Can you work these out from the drawing? Everything is in mm from the part's minimum corner. Coordinates: 2 decimals unless noted, no trailing zeros. Write each loop counter-clockwise with the first axis right and the second up, starting at its lowest first coordinate (ties: lowest second). Pieces come first, ordered by that corner, then holes. Notation, with made-up numbers: M -17.5,28 L 21.5,28 A30 cw 21.5,65 Z; hole C -19,85.5 d2. An arc over 180 degrees is marked long. Write item = value, one per line.
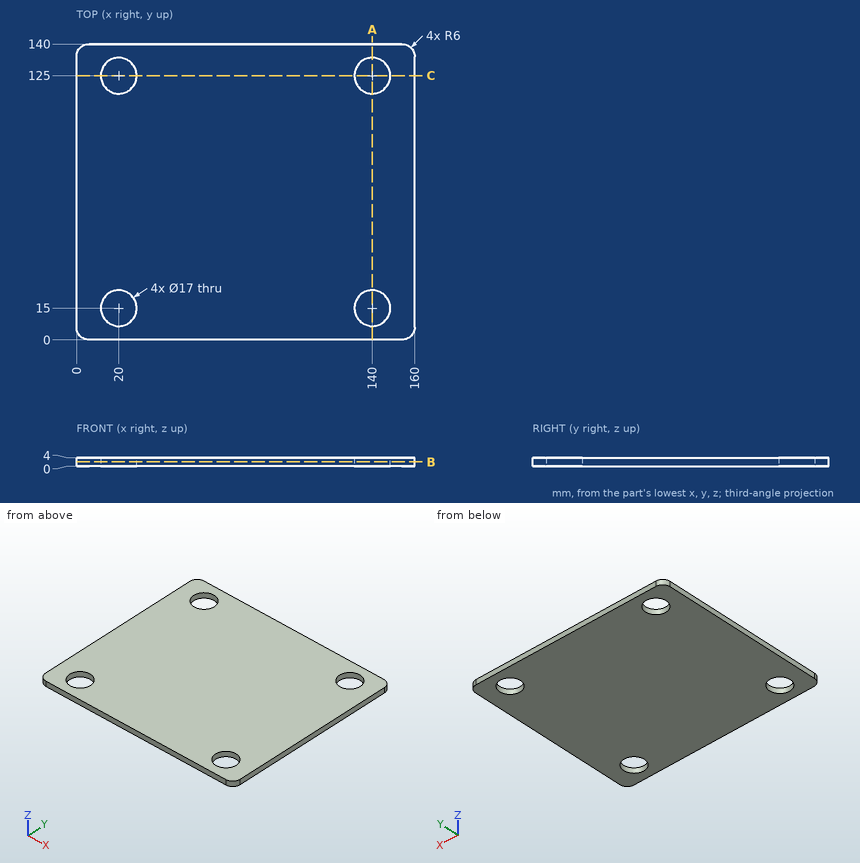
Item 1: Imagine slicing it at C-C (y = 125). Write out the boundary of the cut face in (x, z), and give its area (3 significant figures).
Numbers:
outline = M 0,0 L 11.5,0 L 11.5,4 L 0,4 Z; M 28.5,0 L 131.5,0 L 131.5,4 L 28.5,4 Z; M 148.5,0 L 160,0 L 160,4 L 148.5,4 Z
area = 504 mm²
Item 2: Imagine slicing it at B-B (z = 2.1). Write out the boundary of the cut face in (x, y), and give its area (3 significant figures).
Numbers:
outline = M 0,6 A6 ccw 6,0 L 154,0 A6 ccw 160,6 L 160,134 A6 ccw 154,140 L 6,140 A6 ccw 0,134 Z; hole C 20,15 d17; hole C 20,125 d17; hole C 140,15 d17; hole C 140,125 d17
area = 21,500 mm²
Item 3: If I drill on line 1 along Y through (x, z) = (20, 0.95); line 2 along X through (y, z) = (120.5, 3.25); line 3 along Y through (x, z) = (22, 0.45), over which ranges is the centre line in solid material (lowest first)?
Numbers:
line_1 = 0 to 6.5, 23.5 to 116.5, 133.5 to 140
line_2 = 0 to 12.79, 27.21 to 132.79, 147.21 to 160
line_3 = 0 to 6.74, 23.26 to 116.74, 133.26 to 140
Item 4: I'm going to push a flat-ended pin straight in: P1, Ø10, axis at x = 140, y = 125, coming from the +Z side. Where does the tip first touch, or does it pass through?
Numbers:
P1 = through
Item 5: Imagine slicing it at A-A (x = 140). Write out the boundary of the cut face in (y, z).
Numbers:
outline = M 0,0 L 6.5,0 L 6.5,4 L 0,4 Z; M 23.5,0 L 116.5,0 L 116.5,4 L 23.5,4 Z; M 133.5,0 L 140,0 L 140,4 L 133.5,4 Z
